Build history of the part. All positions in model axes, mm. Round coordinates to 2 decimals unless told otherwise and drop trailing zeros. Write each loop counter-clockwise with the first axis right and the second up, starting at its lowest first coordinate (ties: lowest second). Pieces come first, ordered by that corner, then holes. Notation, with made-up numbers: (21.5, 61) -> (39.5, 61) arc R27 ccw to (39.5, 89) -> close; hole circle Ø11 at (-29.5, 68.25). An arc over 180 degrees is marked (long way). Return JSON: item names as keys, results as strings.
from build123d import *

# Parameters (mm, degrees)
BOSS_EXTRUDE1_DEPTH = 6.6
CUT_EXTRUDE1_DEPTH  = 6.6
CUT_EXTRUDE2_DEPTH  = 1.6
CUT_EXTRUDE3_DEPTH  = 11.6
SKETCH5_W           = 9.5
SKETCH5_H           = 4.05
CUT_EXTRUDE4_DEPTH  = 2
SKETCH6_W           = 0.75
SKETCH6_H           = 40
SKETCH6_W_2         = 55
SKETCH6_H_2         = 0.75
CUT_EXTRUDE5_DEPTH  = 2.6
SKETCH7_W           = 0.6
SKETCH7_H           = 40
SKETCH7_W_2         = 55
SKETCH7_H_2         = 0.6
BOSS_EXTRUDE2_DEPTH = 2.4


with BuildPart() as part:
    # Sketch1 → Boss-Extrude1 (new body)
    with BuildSketch(Plane(origin=(0, 0, 0), x_dir=(1, 0, 0), z_dir=(0, 1, 0))):
        with BuildLine():
            Line((3, 0), (64.1, 0))
            ThreePointArc((64.1, 0), (66.221320344, 0.878679656), (67.1, 3))
            Line((67.1, 3), (67.1, 49))
            ThreePointArc((67.1, 49), (66.221320344, 51.121320344), (64.1, 52))
            Line((64.1, 52), (3, 52))
            ThreePointArc((3, 52), (0.878679656, 51.121320344), (0, 49))
            Line((0, 49), (0, 3))
            ThreePointArc((0, 3), (0.878679656, 0.878679656), (3, 0))
        make_face()
    extrude(amount=BOSS_EXTRUDE1_DEPTH)

    # Sketch2 → Cut-Extrude1 (cut)
    with BuildSketch(Plane(origin=(0, 6.6, 0), x_dir=(1, 0, 0), z_dir=(0, 1, 0))):
        with BuildLine():
            Line((6.05, 3.05), (61.05, 3.05))
            ThreePointArc((61.05, 3.05), (63.171320344, 3.928679656), (64.05, 6.05))
            Line((64.05, 6.05), (64.05, 44.05))
            ThreePointArc((64.05, 44.05), (63.171320344, 46.171320344), (61.05, 47.05))
            Line((61.05, 47.05), (6.05, 47.05))
            ThreePointArc((6.05, 47.05), (3.928679656, 46.171320344), (3.05, 44.05))
            Line((3.05, 44.05), (3.05, 6.05))
            ThreePointArc((3.05, 6.05), (3.928679656, 3.928679656), (6.05, 3.05))
        make_face()
    extrude(amount=-CUT_EXTRUDE1_DEPTH, mode=Mode.SUBTRACT)

    # Sketch3 → Cut-Extrude2 (cut)
    with BuildSketch(Plane(origin=(0, 6.6, 0), x_dir=(1, 0, 0), z_dir=(0, 1, 0))):
        with BuildLine():
            Line((4.65, 51.1), (62.45, 51.1))
            ThreePointArc((62.45, 51.1), (64.394543648, 50.294543648), (65.2, 48.35))
            Line((65.2, 48.35), (65.2, 4.65))
            ThreePointArc((65.2, 4.65), (64.394543648, 2.705456352), (62.45, 1.9))
            Line((62.45, 1.9), (4.65, 1.9))
            ThreePointArc((4.65, 1.9), (2.705456352, 2.705456352), (1.9, 4.65))
            Line((1.9, 4.65), (1.9, 48.35))
            ThreePointArc((1.9, 48.35), (2.705456352, 50.294543648), (4.65, 51.1))
        make_face()
    extrude(amount=-CUT_EXTRUDE2_DEPTH, mode=Mode.SUBTRACT)

    # Sketch4 → Cut-Extrude3 (cut)
    with BuildSketch(Plane(origin=(0, 0, -52), x_dir=(-1, 0, 0), z_dir=(0, 0, -1))):
        with BuildLine():
            Line((-37.16, 5.2), (-29.46, 5.2))
            ThreePointArc((-29.46, 5.2), (-28.823603897, 4.936396103), (-28.56, 4.3))
            Line((-28.56, 4.3), (-28.56, 2.5))
            ThreePointArc((-28.56, 2.5), (-28.823603897, 1.863603897), (-29.46, 1.6))
            Line((-29.46, 1.6), (-37.16, 1.6))
            ThreePointArc((-37.16, 1.6), (-37.796396103, 1.863603897), (-38.06, 2.5))
            Line((-38.06, 2.5), (-38.06, 4.3))
            ThreePointArc((-38.06, 4.3), (-37.796396103, 4.936396103), (-37.16, 5.2))
        make_face()
    extrude(amount=-CUT_EXTRUDE3_DEPTH, mode=Mode.SUBTRACT)

    # Sketch5 → Cut-Extrude4 (cut)
    with BuildSketch(Plane(origin=(0, 5, 0), x_dir=(1, 0, 0), z_dir=(0, 1, 0))):
        with Locations((33.31, 49.075)):
            Rectangle(SKETCH5_W, SKETCH5_H)
    extrude(amount=-CUT_EXTRUDE4_DEPTH, mode=Mode.SUBTRACT)

    # Sketch6 → Cut-Extrude5 (cut)
    with BuildSketch(Plane.XZ):
        with Locations((65.975, -26)):
            Rectangle(SKETCH6_W, SKETCH6_H)
        with Locations((1.125, -26)):
            Rectangle(SKETCH6_W, SKETCH6_H)
        with Locations((33.55, -1.125)):
            Rectangle(SKETCH6_W_2, SKETCH6_H_2)
    extrude(amount=-CUT_EXTRUDE5_DEPTH, mode=Mode.SUBTRACT)

    # Sketch7 → Boss-Extrude2 (add)
    with BuildSketch(Plane(origin=(0, 6.6, 0), x_dir=(1, 0, 0), z_dir=(0, 1, 0))):
        with Locations((1, 26)):
            Rectangle(SKETCH7_W, SKETCH7_H)
        with Locations((33.55, 1)):
            Rectangle(SKETCH7_W_2, SKETCH7_H_2)
        with Locations((66.1, 26)):
            Rectangle(SKETCH7_W, SKETCH7_H)
    extrude(amount=BOSS_EXTRUDE2_DEPTH)


solid = part.part
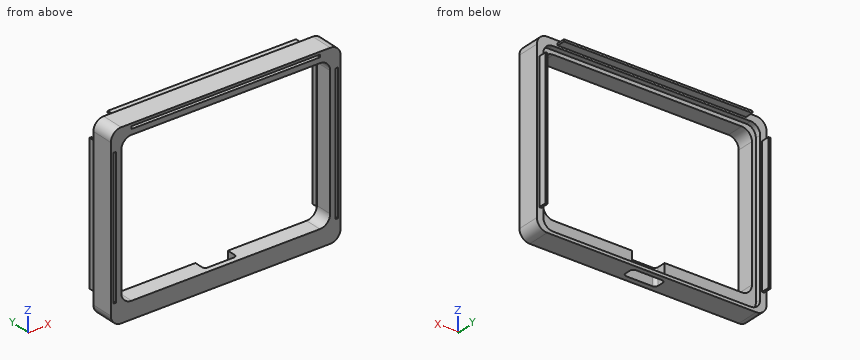
Q1. Saw through at C-C on x = 56. List the corners of the cut face in (y, z).
Verdict:
{"outline": "(0, -52) -> (6.6, -52) -> (6.6, -51.1) -> (5, -51.1) -> (5, -47.05) -> (0, -47.05) -> close; (0, -3.05) -> (5, -3.05) -> (5, -1.9) -> (6.6, -1.9) -> (6.6, -1.3) -> (9, -1.3) -> (9, -0.7) -> (6.6, -0.7) -> (6.6, 0) -> (0, 0) -> (0, -0.75) -> (2.6, -0.75) -> (2.6, -1.5) -> (0, -1.5) -> close"}
Q2. Saw through at B-B on x = 35. List the corners of the cut face in (y, z).
Verdict:
{"outline": "(0, -52) -> (1.6, -52) -> (1.6, -47.05) -> (0, -47.05) -> close; (0, -3.05) -> (5, -3.05) -> (5, -1.9) -> (6.6, -1.9) -> (6.6, -1.3) -> (9, -1.3) -> (9, -0.7) -> (6.6, -0.7) -> (6.6, 0) -> (0, 0) -> (0, -0.75) -> (2.6, -0.75) -> (2.6, -1.5) -> (0, -1.5) -> close; (5.2, -52) -> (6.6, -52) -> (6.6, -51.1) -> (5.2, -51.1) -> close"}
Q3. Saw through at D-D on z = -40.5. List the corners of the cut face in (x, y), then the cut area to 3 significant figures.
Verdict:
{"outline": "(0, 0) -> (0.75, 0) -> (0.75, 2.6) -> (1.5, 2.6) -> (1.5, 0) -> (3.05, 0) -> (3.05, 5) -> (1.9, 5) -> (1.9, 6.6) -> (1.3, 6.6) -> (1.3, 9) -> (0.7, 9) -> (0.7, 6.6) -> (0, 6.6) -> close; (64.05, 0) -> (65.6, 0) -> (65.6, 2.6) -> (66.35, 2.6) -> (66.35, 0) -> (67.1, 0) -> (67.1, 6.6) -> (66.4, 6.6) -> (66.4, 9) -> (65.8, 9) -> (65.8, 6.6) -> (65.2, 6.6) -> (65.2, 5) -> (64.05, 5) -> close", "area": "35.6 mm²"}
Q4. Saw through at A-A on y = 7.5. List the corners of the cut face in (x, z), then the cut area to 3 significant figures.
Verdict:
{"outline": "(0.7, -46) -> (1.3, -46) -> (1.3, -6) -> (0.7, -6) -> close; (6.05, -1.3) -> (61.05, -1.3) -> (61.05, -0.7) -> (6.05, -0.7) -> close; (65.8, -46) -> (66.4, -46) -> (66.4, -6) -> (65.8, -6) -> close", "area": "81.0 mm²"}
Q5. Pin check, flat tips, straight feed: pin 1 Ø0.8 at (x, y) = (1, 1.5) entering from -Z; pin 2 Ø0.6 at (y, z) = (1.5, -1.5) entering from +X; pin 3 Ø1.9 at (x, y) = (29, 8.5) entering from -Z. Stop position of each tip, or through.
Verdict:
{"pin 1": "stops at z = -51.54", "pin 2": "stops at x = 66.85", "pin 3": "stops at z = -1.3"}
Q6. Wall check: L1, parallel to Z at x = 26, y = 2.5; L2, parallel to X at y = 2, z = -23; L3, parallel to X at y = 8.5, z = -14. Give the ranges that are in metal, low to high.
Verdict:
{"L1": "z = -52 to -47.05, -3.05 to -1.5, -0.75 to 0", "L2": "x = 0 to 0.75, 1.5 to 3.05, 64.05 to 65.6, 66.35 to 67.1", "L3": "x = 0.7 to 1.3, 65.8 to 66.4"}
